The figure shows three views and two pictorial views of one solid part (mm, origin at its lowest corner). Answer the questions. A direction names the side the tool comes from. Round coordinates to 2 decimals unless told otherwise and drop trailing zeros. Write each loop counter-clockwise with the first axis right and the second up, starting at its lowest first coordinate (ties: lowest second). Pieces come first, ordered by that corner, then holes. Notation, with made-up numbers: (10, 18) -> (54, 18) arc R12 ccw to (54, 34) -> close; hole circle Ø5 at (-23.5, 6.25). An arc over 180 degrees is marked (long way). One line per item, written item: value.
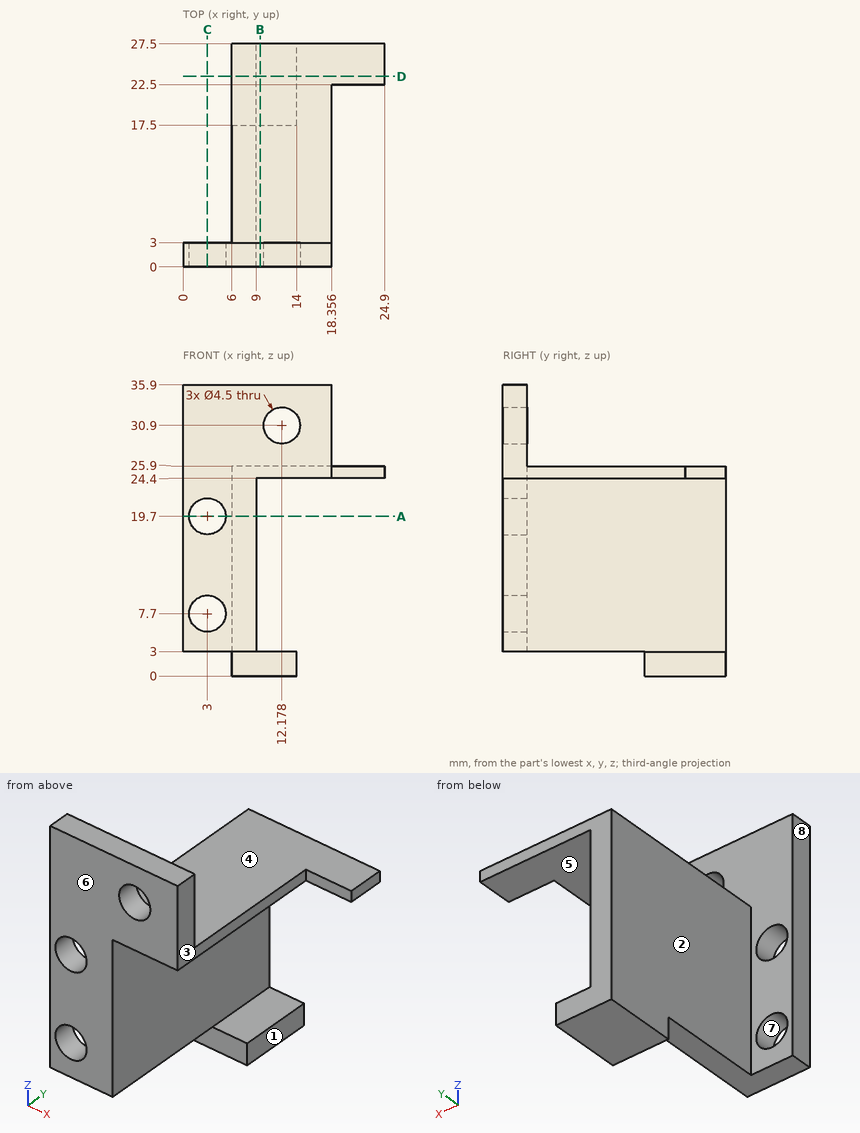
(1) Find section B-B on x = 9.5. Give the vertices of the cut face in (y, z).
Reported:
outline: (0, 24.4) -> (27.5, 24.4) -> (27.5, 25.9) -> (3, 25.9) -> (3, 35.9) -> (0, 35.9) -> close; (17.5, 0) -> (27.5, 0) -> (27.5, 3) -> (17.5, 3) -> close
(2) Find section C-C on x = 3. Give the vertices of the cut face in (y, z).
Reported:
outline: (0, 3) -> (3, 3) -> (3, 5.45) -> (0, 5.45) -> close; (0, 9.95) -> (3, 9.95) -> (3, 17.45) -> (0, 17.45) -> close; (0, 21.95) -> (3, 21.95) -> (3, 35.9) -> (0, 35.9) -> close
(3) Consider probe 1 along Z at (x, y) = (3, 1.3); probe 2 along X at (y, z) = (1.05, 19.7); probe 3 along X at (y, z) = (16, 15). Determine where each line is inside the solid, lowest interval first.
Reported:
probe 1: z = 3 to 5.45, 9.95 to 17.45, 21.95 to 35.9
probe 2: x = 0 to 0.75, 5.25 to 9
probe 3: x = 6 to 9
(4) Find section A-A on z = 19.7. Give the vertices of the cut face in (x, y).
Reported:
outline: (0, 0) -> (0.75, 0) -> (0.75, 3) -> (0, 3) -> close; (5.25, 0) -> (9, 0) -> (9, 27.5) -> (6, 27.5) -> (6, 3) -> (5.25, 3) -> close
(5) For a pull along X with two mould halves and no side action, classify the marked faces 6, 7 and 8 as pulls with the +X half, pulls with the -X half, needs draft (parallel to the pull), parting line crosses it, or undercut.
Reported:
face 6: needs draft
face 7: undercut
face 8: pulls with the -X half
(6) A tool of negligible diameter and unlimited length cuts with its end or side. For the marked faces 1, 2, 3, 4 and 5, from which of +Z, -Z, +X, -X, +Y, -Y can it reach the whole face along a straight path? Write none if from no direction.
Reported:
face 1: -Z, +X, +Y, -Y
face 2: +Z, -Z, -X, +Y
face 3: +Z, -Z, +X, -Y
face 4: +Z, +X, -X, +Y
face 5: +X, +Y, -Y
(7) Flat-ended cylindrical pins translate along their axes: pin 1 Ø12.5 at (x, y) = (20.5, 20) entering from -Z; pin 2 Ø1.5 at (y, z) = (23.5, 2) entering from +X; pin 3 Ø7 at (x, z) = (3, 7.7) entering from +Y; pin 4 Ø0.9 at (x, z) = (9, 2) entering from -Y. Find the tip coordinate at first contact, or state that the pin passes through.
Reported:
pin 1: stops at z = 24.4
pin 2: stops at x = 14
pin 3: stops at y = 27.5
pin 4: stops at y = 17.5
(8) Find section D-D on y = 23.5. Give the vertices of the cut face in (x, z).
Reported:
outline: (6, 0) -> (14, 0) -> (14, 3) -> (9, 3) -> (9, 24.4) -> (24.9, 24.4) -> (24.9, 25.9) -> (6, 25.9) -> close
